Design review of the part built by this model. Coordinates are the model's own, in mm. Coordinates: 2 decimals unless noted, no trailing zeros. Order: outer loops, then holes, each group sorted by start corner. A loop starts at its lowest first (then second) coordinate and runs counter-clockwise, first axis right, second up. Notation, with made-up numbers: M 73.5,52 L 85.5,52 A12 cw 85.5,70 Z; hole C 64.25,-38.75 d9. An arc over 180 degrees is marked long. Answer as a JSON object with one key per item and string values.
from build123d import *

# Parameters (mm, degrees)
SKETCH7_W          = 172
SKETCH7_H          = 149
BASE_FLANGE2_DEPTH = 10
SKETCH8_R          = 6
SKETCH8_R_2        = 10
CUT_EXTRUDE1_DEPTH = 200.974998437


# Sheet-metal steps are written as plain solids
with BuildPart() as part:
    # Sketch7 → Base-Flange2 (new body)
    with BuildSketch(Plane(origin=(0, 0, 0), x_dir=(1, 0, 0), z_dir=(0, 1, 0))):
        with Locations((47, 74.5)):
            Rectangle(SKETCH7_W, SKETCH7_H)
    extrude(amount=-BASE_FLANGE2_DEPTH)

    # Sketch8 → Cut-Extrude1 (cut, through all)
    with BuildSketch(Plane(origin=(0, 0, 0), x_dir=(1, 0, 0), z_dir=(0, 1, 0))):
        with Locations(Location((9, 120.5, 0), (0, 0, 270))):
            Circle(SKETCH8_R)
        with Locations(Location((85, 120.5, 0), (0, 0, 270))):
            Circle(SKETCH8_R)
        with Locations(Location((9, 28.5, 0), (0, 0, 270))):
            Circle(SKETCH8_R)
        with Locations(Location((47, 74.5, 0), (0, 0, 270))):
            Circle(SKETCH8_R_2)
        with Locations(Location((85, 28.5, 0), (0, 0, 270))):
            Circle(SKETCH8_R)
    extrude(amount=-CUT_EXTRUDE1_DEPTH, mode=Mode.SUBTRACT)


solid = part.part
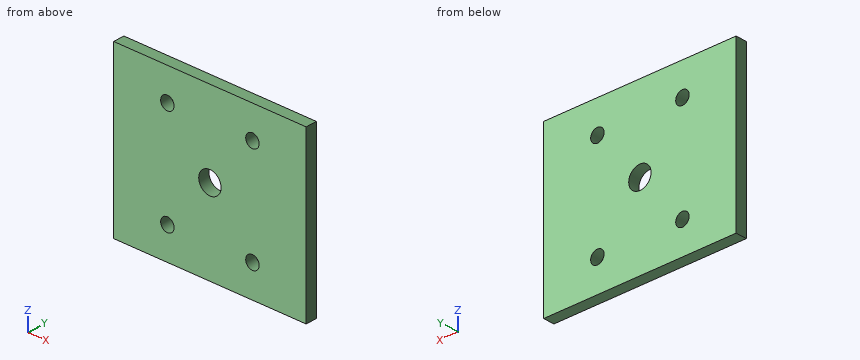
1) Add section D-D (y = -3.25). State the section outline as (x, z) points, and give its area (3 significant figures).
Taken from the geometry:
{"outline": "M -39,-149 L 133,-149 L 133,0 L -39,0 Z; hole C 9,-120.5 d12; hole C 9,-28.5 d12; hole C 47,-74.5 d20; hole C 85,-120.5 d12; hole C 85,-28.5 d12", "area": "24,900 mm2"}
2) Add section A-A (z = -74.5). State the section outline as (x, y) points, and give its area (3 significant figures).
Taken from the geometry:
{"outline": "M -39,-10 L 37,-10 L 37,0 L -39,0 Z; M 57,-10 L 133,-10 L 133,0 L 57,0 Z", "area": "1,520 mm2"}
3) Insertion check: pin 1 Ø9.5 at (x, z) = (85, -120.5) entering from -Y. The pin has a flat end and moves straight along its axis. Give the tip position at first contact, or say it passes through.
Taken from the geometry:
{"pin 1": "passes through"}
4) To check wall thickness, follow L1, parallel to X at y = -5, z = -120.5; L2, parallel to Z at x = 81, y = -7; L3, parallel to X at y = -4, z = -116. State the ranges of each line that lie inside material, in increasing order.
Taken from the geometry:
{"L1": "x = -39 to 3, 15 to 79, 91 to 133", "L2": "z = -149 to -124.97, -116.03 to -32.97, -24.03 to 0", "L3": "x = -39 to 5.03, 12.97 to 81.03, 88.97 to 133"}
5) Add section B-B (x = 9). State the section outline as (y, z) points, and give its area (3 significant figures).
Taken from the geometry:
{"outline": "M -10,-149 L 0,-149 L 0,-126.5 L -10,-126.5 Z; M -10,-114.5 L 0,-114.5 L 0,-34.5 L -10,-34.5 Z; M -10,-22.5 L 0,-22.5 L 0,0 L -10,0 Z", "area": "1,250 mm2"}
6) Add section C-C (z = -28.5). State the section outline as (x, y) points.
Taken from the geometry:
{"outline": "M -39,-10 L 3,-10 L 3,0 L -39,0 Z; M 15,-10 L 79,-10 L 79,0 L 15,0 Z; M 91,-10 L 133,-10 L 133,0 L 91,0 Z"}
